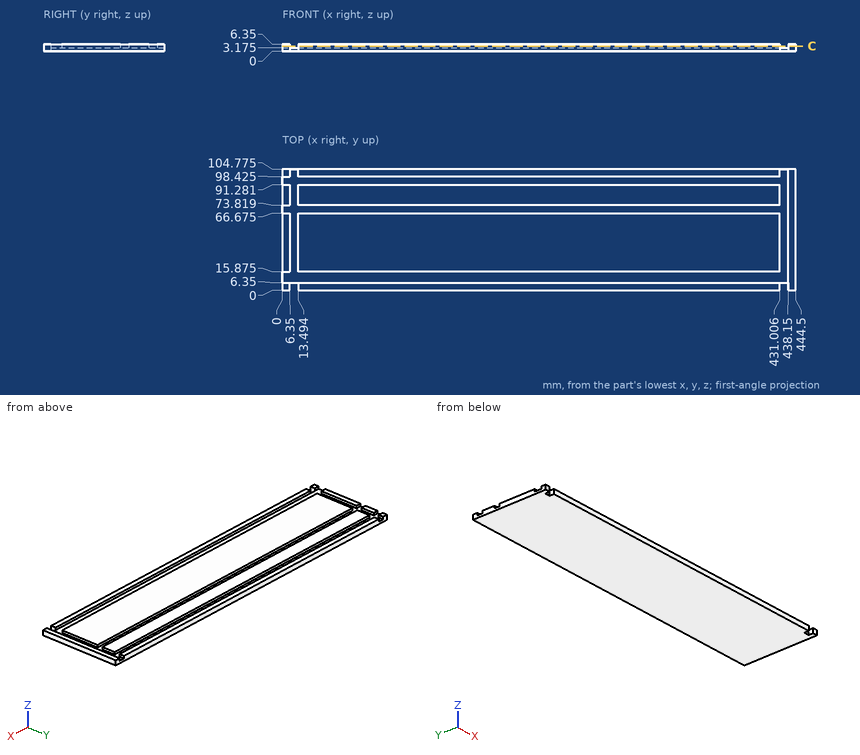
Answer from the drawing. Dimensions are ordinates in mm from the lowest x, y and z of the part. Coordinates: 2 decimals unless noted, no trailing zeros.
Q1. Consider probe 1 along X at (y, z) = (80, 4.75); probe 2 along X at (y, z) = (94, 3.5); probe 3 along Z at (x, y) = (300.5, 67.5) (1 decimal). Determine where each line is inside the solid, lowest interval first.
Q2. The part is cut by section C-C on z = 4.5. Give the number of separate pieces and of enclosed holes in the cut face, and give its area (3 significant figures).
Q3. This flat-tipped pin is pushed along its axis until it touches: pin 1 Ø1.6 at (x, z) = (9, 1.5) entering from -Y. Where does it stop, or does it pass through?
Results below:
1. probe 1: x = 0 to 6.35, 13.49 to 431.01, 438.15 to 444.5
1. probe 2: x = 438.15 to 444.5
1. probe 3: z = 0 to 3.2
2. separate pieces: 9
2. enclosed holes: 0
2. area: 35,000 mm2
3. pin 1: stops at y = 6.35
